Print and shaded views of the part. All mm, measured from the part's lowest x, y and z. A direction names the side the tool comes from. Round coordinates to 2 decimals unless told otherwise and drop trailing zeros. Loops run counter-clockwise (first coordinate to the right, second up) from the corner with the lowest first, then second, coordinate; pieces in that order, holes last. Notation, with made-up numbers: (32.25, -11) -> (42.25, -11) arc R18 ccw to (42.25, 16) -> close; hole circle Ø2 at (-7, -4). An arc over 180 degrees is marked (long way). Use a Markdown table: item, result.
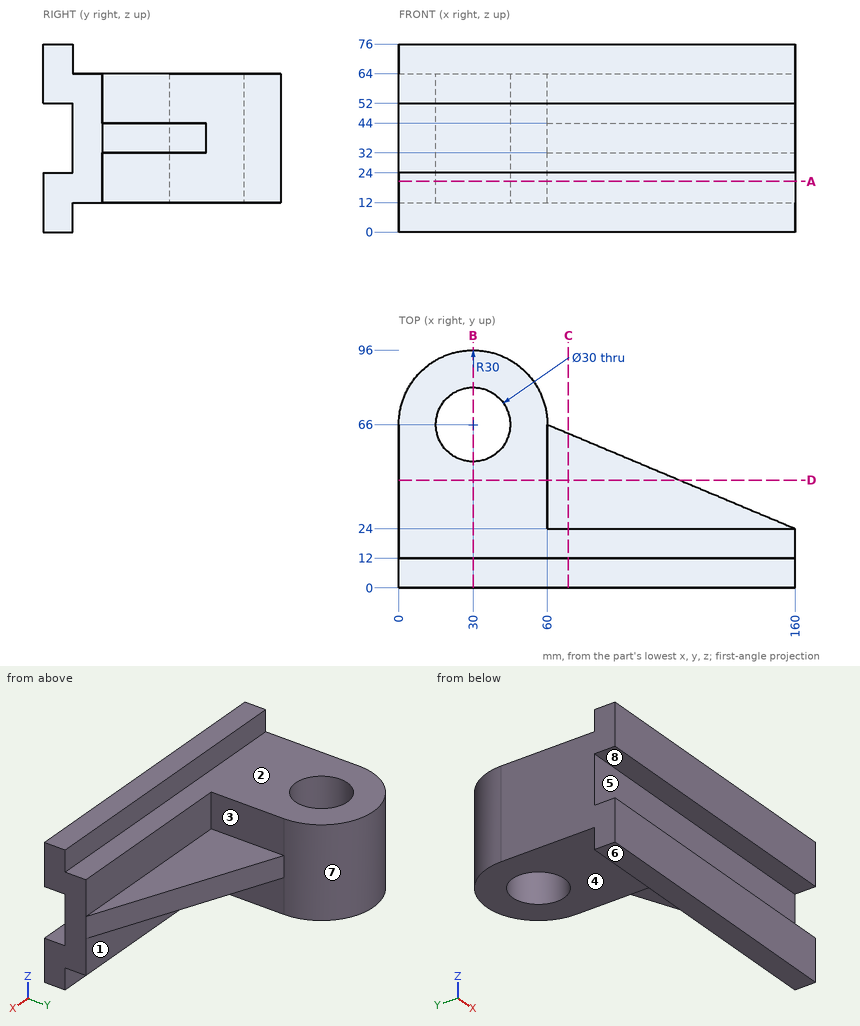
Q1. Flat gauge pins, fed straight in: pin 1 (22 mm diameter, centred on y = 40, z = 56, fed in from +X); pin 2 (16 mm diameter, centred on x = 131, z = 52.5, fed in from +Y); pin 3 (14 mm diameter, centred on x = 99.5, z = 42.5, fed in from -Y). Where does each tip first touch, or does it go through?
Results list:
| item | result |
|---|---|
| pin 1 | stops at x = 60 |
| pin 2 | stops at y = 24 |
| pin 3 | stops at y = 12 |
Q2. Band-saw the part on B-B, the plane x = 30. Give the cut face in (y, z).
Results list:
| item | result |
|---|---|
| outline | (0, 0) -> (12, 0) -> (12, 12) -> (51, 12) -> (51, 64) -> (12, 64) -> (12, 76) -> (0, 76) -> (0, 52) -> (12, 52) -> (12, 24) -> (0, 24) -> close; (81, 12) -> (96, 12) -> (96, 64) -> (81, 64) -> close |
Q3. Band-saw the part on A-A, the plane z = 20.5. Give the cut face in (x, y).
Results list:
| item | result |
|---|---|
| outline | (0, 0) -> (160, 0) -> (160, 24) -> (60, 24) -> (60, 66) arc R30 ccw to (0, 66) -> close; hole circle Ø30 at (30, 66) |
Q4. Band-saw the part on C-C, the plane x = 68.5. Give the cut face in (y, z).
Results list:
| item | result |
|---|---|
| outline | (0, 0) -> (12, 0) -> (12, 12) -> (24, 12) -> (24, 32) -> (62.43, 32) -> (62.43, 44) -> (24, 44) -> (24, 64) -> (12, 64) -> (12, 76) -> (0, 76) -> (0, 52) -> (12, 52) -> (12, 24) -> (0, 24) -> close |
Q5. Band-saw the part on D-D, the plane y = 43.5. Give the cut face in (x, z).
Results list:
| item | result |
|---|---|
| outline | (0, 12) -> (60, 12) -> (60, 32) -> (113.57, 32) -> (113.57, 44) -> (60, 44) -> (60, 64) -> (0, 64) -> close |
Q6. Drill centre lines: L1, parallel to Y at x = 30, z = 30.5; L2, parallel to Z at x = 34, y = 83; L3, parallel to X at y = 38, z = 23.5. Where is each one in solid material? Low to high. Write a range as from..to.
Results list:
| item | result |
|---|---|
| L1 | y = 12..51, 81..96 |
| L2 | z = 12..64 |
| L3 | x = 0..60 |
Q7. Pull direction Z, two halves, no side cores. Call the marked faces 5, 6, 7 and 8: released by +Z, released by -Z, zero draft, split by the parting line, or undercut.
Results list:
| item | result |
|---|---|
| face 5 | undercut |
| face 6 | released by -Z |
| face 7 | zero draft |
| face 8 | undercut |
Q8. Tool access for the marked faces 1, 2, 3 and 4: list every direction of +Z, -Z, +X, -X, +Y, -Y with a clear straight run to the whole face (end or side of a thin tool).
Results list:
| item | result |
|---|---|
| face 1 | -Z, +X, +Y |
| face 2 | +Z, +X, -X, +Y |
| face 3 | +Z, +X, +Y |
| face 4 | -Z, +X, -X, +Y |
